```python
from build123d import *

# Parameters (mm, degrees)
BOSS_EXTRUDE1_DEPTH      = 18.5
SKETCH2_R                = 1.25
CUT_EXTRUDE1_DEPTH       = 18.5
SKETCH3_R                = 1.25
BOSS_EXTRUDE2_DEPTH      = 2.5
BOSS_EXTRUDE2_DEPTH_BACK = 2.5


with BuildPart() as part:
    # Sketch1 → Boss-Extrude1 (new body)
    with BuildSketch(Plane(origin=(0, 0, 0), x_dir=(1, 0, 0), z_dir=(0, 1, 0))):
        Polygon((1.156221884, 1.289632101), (-0.538743219, 1.646133574), (-1.694965103, 0.356501473), (-1.156221884, -1.289632101), (0.538743219, -1.646133574), (1.694965103, -0.356501473), align=None)
    extrude(amount=BOSS_EXTRUDE1_DEPTH)

    # Sketch2 → Cut-Extrude1 (cut)
    with BuildSketch(Plane(origin=(0, 18.5, 0), x_dir=(1, 0, 0), z_dir=(0, 1, 0))):
        Circle(SKETCH2_R)
    extrude(amount=-CUT_EXTRUDE1_DEPTH, mode=Mode.SUBTRACT)

    # Sketch3 → Boss-Extrude2 (add, two sides)
    with BuildSketch(Plane.XZ) as boss_extrude2_sk:
        Circle(SKETCH3_R)
    extrude(amount=BOSS_EXTRUDE2_DEPTH)
    extrude(boss_extrude2_sk.sketch, amount=-BOSS_EXTRUDE2_DEPTH_BACK)


solid = part.part
```
Here's how the part is built. I have some questions about the finished solid (model axes, mm). A direction names the side the tool comes from. Round coordinates to 2 decimals unless told otherwise and drop trailing zeros. Order: outer loops, then holes, each group sorted by start corner. A loop starts at its lowest first (then second) coordinate and runs counter-clockwise, first axis right, second up. Notation, with made-up numbers: (28.25, 23) -> (80.25, 23) arc R33 cw to (80.25, 56) -> close; hole circle Ø3 at (81.5, 28.5). An arc over 180 degrees is marked (long way). Use a Markdown table: item, result. Add a question column.
(1) I need wall thicknesses on line 1 along Y through (x, z) = (0.7, 0.05); line 2 along Y through (x, z) = (-1.2, -0.8); line 3 along Z through (x, y) = (1, 9). Which ranges of each line are inside material? Lowest first, please.
(2) For pin 1 Ø1.5 at (x, y) = (-1, 11.5) entering from +Z; pin 2 Ø0.8 at (x, z) = (0, -0.5) entering from +Y, each with a flat end and sliding along its axis, tell me the tip position at first contact or that it passes through.
(3) Suppose I cut it at A-A, the plane z = 0.9. Please give me the cut outline in (x, y), and give its area (3 significant figures).
(4) For faces 1 (the face through (-0.27, 10.61, 1.22)), 2 (the face through (-1, 0, 1)), 3 (the face through (-1, 18.5, 1)), which set-ups out of +Z, -Z, +X, -X, +Y, -Y let a thin tool reach every point of the face, with its end or its side?
(5) If we mould it in two halves opening along X, with no side actions, what happens to faces 4 (the face through (1.429, 9.12, -0.455)), 5 (the face through (0, -2.5, 0)), 6 (the face through (0, 2.5, 0))? For each: released by +X, released by -X, zero draft, split by the parting line, or undercut.
(6) Suppose I cut it at B-B, the plane x = 0. Please give me the cut outline in (y, z), and give its area (3 significant figures).
Verdict:
| question | item | result |
|---|---|---|
| 1 | line 1 | -2.5 to 2.5 |
| 1 | line 2 | 0 to 18.5 |
| 1 | line 3 | -1.32 to -0.75, 0.75 to 1.13 |
| 2 | pin 1 | z = 1.48 |
| 2 | pin 2 | y = 2.5 |
| 3 | outline | (-1.28, 0) -> (-0.87, 0) -> (-0.87, -2.5) -> (0.87, -2.5) -> (0.87, 0) -> (1.21, 0) -> (1.21, 18.5) -> (0.87, 18.5) -> (0.87, 2.5) -> (-0.87, 2.5) -> (-0.87, 18.5) -> (-1.28, 18.5) -> close |
| 3 | area | 22.7 mm2 |
| 4 | face 1 | +Y |
| 4 | face 2 | -Y |
| 4 | face 3 | +Z, -Z, +X, -X, +Y |
| 5 | face 4 | released by +X |
| 5 | face 5 | zero draft |
| 5 | face 6 | undercut |
| 6 | outline | (-2.5, -1.25) -> (0, -1.25) -> (0, -1.53) -> (18.5, -1.53) -> (18.5, -1.25) -> (2.5, -1.25) -> (2.5, 1.25) -> (18.5, 1.25) -> (18.5, 1.53) -> (0, 1.53) -> (0, 1.25) -> (-2.5, 1.25) -> close |
| 6 | area | 23.0 mm2 |
